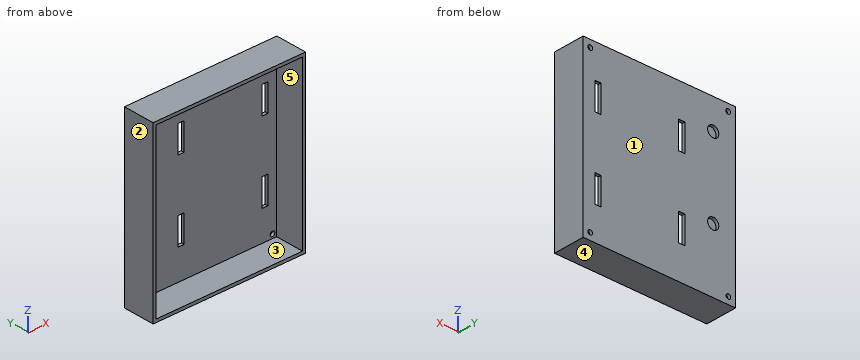
Autodesk Inventor part; units mm, degrees
ref_plane "YZ Plane" through (0, 0, 0) normal (1, 0, 0) x (0, 1, 0)
ref_plane "XZ Plane" through (0, 0, 0) normal (0, 1, 0) x (-1, 0, 0)
ref_plane "XY Plane" through (0, 0, 0) normal (0, 0, 1) x (1, 0, 0)
sketch "Sketch1" plane through (0, 0, 0) normal (0, 1, 0) x (-1, 0, 0)
  line L0 (-58.4836, 42.7915) -> (-27.4836, 42.7915) construction
  line L1 (-27.4836, 42.7915) -> (-27.4836, 11.7915) construction
  line L2 (-27.4836, 11.7915) -> (-58.4836, 11.7915) construction
  line L3 (-58.4836, 11.7915) -> (-58.4836, 20.5915) construction
  line L4 (-58.4836, 42.7915) -> (-27.4836, 11.7915) construction
  line L5 (-27.4836, 42.7915) -> (-58.4836, 11.7915) construction
  line L6 (-58.4836, 3.6103) -> (-27.4836, 3.6103) construction
  line L7 (-27.4836, 3.6103) -> (-27.4836, -27.2085) construction
  line L8 (-27.4836, -27.2085) -> (-58.4836, -27.2085) construction
  line L9 (-58.4836, -27.2085) -> (-58.4836, -18.4991) construction
  line L10 (-58.4836, 3.6103) -> (-27.4836, -27.2085) construction
  line L11 (-20.4336, 38.5415) -> (2.0664, 38.5415) construction
  line L12 (2.0664, 38.5415) -> (2.0664, 16.0415) construction
  line L13 (2.0664, 16.0415) -> (-20.4336, 16.0415) construction
  line L14 (-20.4336, 16.0415) -> (-20.4336, 38.5415) construction
  line L15 (-20.4336, 38.5415) -> (2.0664, 16.0415) construction
  line L16 (2.0664, 38.5415) -> (-20.4336, 16.0415) construction
  line L17 (-20.5481, -0.4585) -> (2.0664, -0.4585) construction
  line L18 (2.0664, -0.4585) -> (2.0664, -22.9585) construction
  line L19 (2.0664, -22.9585) -> (-20.5481, -22.9585) construction
  line L20 (-20.5481, -22.9585) -> (-20.5481, -0.4585) construction
  line L21 (-20.5481, -0.4585) -> (2.0664, -22.9585) construction
  line L22 (2.0664, -0.4585) -> (-20.5481, -22.9585) construction
  line L23 (3.5664, -29.3085) -> (-60.5836, -29.3085) construction
  line L24 (-60.5836, -29.3085) -> (-60.5836, 44.8915) construction
  line L25 (-60.5836, 44.8915) -> (-64.5836, 44.8915) construction
  line L26 (-64.5836, 44.8915) -> (-64.5836, 48.8915)
  line L27 (-64.5836, 48.8915) -> (-60.5836, 48.8915)
  line L28 (-60.5836, 48.8915) -> (-60.5836, 44.8915) construction
  line L29 (-60.5836, -29.3085) -> (-64.5836, -29.3085) construction
  line L30 (-64.5836, -29.3085) -> (-64.5836, -33.3085)
  line L31 (-64.5836, -33.3085) -> (-60.5836, -33.3085)
  line L32 (-60.5836, -33.3085) -> (-60.5836, -29.3085) construction
  line L33 (3.5664, -29.3085) -> (7.5664, -29.3085) construction
  line L34 (7.5664, -29.3085) -> (7.5664, -33.3085)
  line L35 (7.5664, -33.3085) -> (3.5664, -33.3085)
  line L36 (3.5664, -33.3085) -> (3.5664, -29.3085) construction
  line L37 (3.5664, 44.8915) -> (7.5664, 44.8915) construction
  line L38 (7.5664, 44.8915) -> (7.5664, 48.8915)
  line L39 (7.5664, 48.8915) -> (3.5664, 48.8915)
  line L40 (3.5664, 48.8915) -> (3.5664, 44.8915) construction
  circle A0 centre (5.4519, 46.9805) radius 1.15
  circle A1 centre (-62.5836, 46.8915) radius 1.15
  circle A2 centre (-62.5836, -31.3085) radius 1.15
  circle A3 centre (5.5664, -31.3085) radius 1.15
  line L41 (3.5664, 48.8915) -> (-60.5836, 48.8915)
  line L42 (-64.5836, 44.8915) -> (-64.5836, -29.3085)
  line L43 (-60.5836, -33.3085) -> (3.5664, -33.3085)
  line L44 (7.5664, -29.3085) -> (7.5664, 44.8915)
  line L45 (3.5664, 44.8915) -> (-60.5836, 44.8915) construction
  line L46 (3.5664, 44.8915) -> (3.5664, -29.3085) construction
  line L47 (-57.2836, 33.9915) -> (-60.2836, 33.9915)
  line L48 (-60.2836, 33.9915) -> (-60.2836, 20.5915)
  line L49 (-60.2836, 20.5915) -> (-57.2836, 20.5915)
  line L50 (-57.2836, 20.5915) -> (-57.2836, 33.9915)
  line L51 (-57.2836, -5.0991) -> (-60.2836, -5.0991)
  line L52 (-60.2836, -5.0991) -> (-60.2836, -18.4991)
  line L53 (-60.2836, -18.4991) -> (-57.2836, -18.4991)
  line L54 (-57.2836, -18.4991) -> (-57.2836, -5.0991)
  line L55 (-58.4836, 20.5915) -> (-58.4836, 33.9915) construction
  line L56 (-58.4836, 33.9915) -> (-58.4836, 42.7915) construction
  line L57 (-58.4836, -5.0991) -> (-58.4836, 3.6103) construction
  line L58 (-58.4836, -18.4991) -> (-58.4836, -5.0991) construction
  line L59 (-62.5836, 46.8915) -> (-60.5836, 46.8915) construction
  line L60 (-62.5836, 46.8915) -> (-62.5836, 44.8915) construction
  line L61 (-62.5836, 46.8915) -> (-64.5836, 46.8915) construction
  line L62 (-62.5836, 46.8915) -> (-62.5836, 48.8915) construction
  line L63 (-64.5836, -31.3085) -> (-62.5836, -31.3085) construction
  line L64 (-62.5836, -31.3085) -> (-60.5836, -31.3085) construction
  line L65 (-62.5836, -31.3085) -> (-62.5836, -29.3085) construction
  line L66 (-62.5836, -31.3085) -> (-62.5836, -33.3085) construction
  line L67 (5.5664, 46.8915) -> (3.5664, 46.8915) construction
  line L68 (5.5664, 46.8915) -> (7.5664, 46.8915) construction
  line L69 (5.5664, 46.8915) -> (5.5664, 44.8915) construction
  line L70 (5.5664, 44.8915) -> (5.5664, 46.8915) construction
  line L71 (5.5664, 46.8915) -> (5.5664, 48.8915) construction
  line L72 (5.5664, -31.3085) -> (5.5664, -33.3085) construction
  line L73 (5.5664, -31.3085) -> (3.5664, -31.3085) construction
  line L74 (5.5664, -31.3085) -> (5.5664, -29.3085) construction
  line L75 (5.5664, -31.3085) -> (7.5664, -31.3085) construction
  circle A4 centre (-1.9336, 35.5415) radius 2.75
  circle A5 centre (-1.9336, -3.4585) radius 2.75
  line L76 (-1.9336, 35.5415) -> (-1.9336, 38.5415) construction
  line L77 (-1.9336, 35.5415) -> (2.0664, 35.5415) construction
  line L78 (-1.9336, -3.4585) -> (2.0664, -3.4585) construction
  line L79 (-1.9336, -3.4585) -> (-1.9336, -0.4585) construction
  line L80 (-15.9336, 33.9915) -> (-18.9336, 33.9915)
  line L81 (-18.9336, 33.9915) -> (-18.9336, 20.5915)
  line L82 (-18.9336, 20.5915) -> (-15.9336, 20.5915)
  line L83 (-15.9336, 20.5915) -> (-15.9336, 33.9915)
  line L84 (-15.9336, -5.0085) -> (-18.9336, -5.0085)
  line L85 (-18.9336, -5.0085) -> (-18.9336, -18.4085)
  line L86 (-18.9336, -18.4085) -> (-15.9336, -18.4085)
  line L87 (-15.9336, -18.4085) -> (-15.9336, -5.0085)
  line L88 (9.0664, 50.3915) -> (-66.0836, 50.3915)
  line L89 (-66.0836, 50.3915) -> (-66.0836, -34.8085)
  line L90 (-66.0836, -34.8085) -> (9.0664, -34.8085)
  line L91 (9.0664, -34.8085) -> (9.0664, 50.3915)
  point P0 (-89.8981, -75.7195)
  dimension "d0" = 22.5
  dimension "d5" = 31
  dimension "d7" = 22.5
  dimension "d11" = 4
  dimension "d12" = 72.15
  dimension "d13" = 82.2
  dimension "d14" = 2.3
  dimension "d15" = 31
  dimension "d16" = 5.5
  dimension "d17" = 5.5
  dimension "d18" = 10.35
  dimension "d19" = 10.35
  dimension "d20" = 6.1
  dimension "d21" = 6.1
  dimension "d22" = 6.1
  dimension "d23" = 6.1
  dimension "d24" = 3
  dimension "d25" = 13.4
  dimension "d26" = 1.2
  dimension "d27" = 8.1812
  dimension "d28" = 16.5
  dimension "d29" = 5.5
  dimension "d30" = 5.5
  dimension "d31" = 3
  dimension "d32" = 4
  dimension "d33" = 1.5
  dimension "d34" = 4.55
  dimension "d35" = 4.55
  dimension "d36" = 4.55
  dimension "d37" = 1.5
  dimension "d38" = 1.5
  dimension "d39" = 1.5
  dimension "d40" = 1.5
extrude "Edges" add sketch "Sketch1" against normal blind 14 contours L91 L90 L89 L88
extrude "Surface" add sketch "Sketch1" along normal blind 1.5 contours L26 L27 L41 L39 L38 L44 L34 L35 L43 L31 L30 L42 | L91 L90 L89 L88
properties part number "CameraBoardCover" material "NylonD2W"
Design review of the part built by this model. Coordinates are the model's own, in mm. Face numbers are marked on the shaded views. A direction names the side the tool comes from. Coordinates: 2 decimals unless noted, no trailing zeros. Order: outer loops, then holes, each group sorted by start corner. A loop starts at its lowest first (then second) coordinate and runs counter-clockwise, first axis right, second up. Notation, with made-up numbers: (-3.75, 78.25) - (28.25, 78.25) arc R32 cw to (28.25, 106.25) - close; hole circle Ø5 at (-18.5, 74.5). An arc over 180 degrees is marked (long way). Answer in a Markdown table with one row per item.
(1) Clearance check with flat-ended pins moving along their axes: pin 1 (10 mm diameter, centred on x = 19, z = 30, fed in from -Y); pin 2 (3 mm diameter, centred on x = 62.58, z = 46.89, fed in from +Y). State where each tip first meets the part, or that it passes through.
Checked values:
| item | result |
|---|---|
| pin 1 | y = 0 |
| pin 2 | y = 1.5 |
(2) Consider section A-A on z = -2. State the section outline as (x, y) points, plus the area to 3 significant figures.
Checked values:
| item | result |
|---|---|
| outline | (-9.07, -14) - (-7.57, -14) - (-7.57, 0) - (-0.4, 0) - (-0.4, 1.5) - (-9.07, 1.5) - close; (4.26, 0) - (64.58, 0) - (64.58, -14) - (66.08, -14) - (66.08, 1.5) - (4.26, 1.5) - close |
| area | 148 mm^2 |
(3) The part is to be moulded in two halves that separate along X. For the marked faces 1, 2 and 3, say which applies: released by +X, released by -X, zero draft, split by the parting line, or undercut.
Checked values:
| item | result |
|---|---|
| face 1 | zero draft |
| face 2 | released by -X |
| face 3 | undercut |
(4) Wall thickness on line 1 along X through (y, z) = (-10.75, 21.5); line 2 along Z through (x, y) = (-6, -3.5); line 3 along Y through (x, z) = (17, 17.5): over which ranges is each line inside the solid? List them lowest first. Write a range as from..to.
Checked values:
| item | result |
|---|---|
| line 1 | -9.07..-7.57, 64.58..66.08 |
| line 2 | -34.81..-33.31, 48.89..50.39 |
| line 3 | 0..1.5 |
(5) For the marked faces 4 and 5, list the 3-axis set-ups (+Z, -Z, +X, -X, +Y, -Y) from which the entire face can be reached by the end or side of a thin tool; tool diameter is ignored.
Checked values:
| item | result |
|---|---|
| face 4 | -Z, +X, -X, +Y, -Y |
| face 5 | -Y |
(6) Consider section C-C on x = 38. State the section outline as (y, z) points, plus the area to 3 significant figures.
Checked values:
| item | result |
|---|---|
| outline | (-14, -34.81) - (1.5, -34.81) - (1.5, 50.39) - (-14, 50.39) - (-14, 48.89) - (0, 48.89) - (0, -33.31) - (-14, -33.31) - close |
| area | 170 mm^2 |
(7) Consider section B-B on y = -9.25. State the section outline as (x, z) points, plus the area to 3 significant figures.
Checked values:
| item | result |
|---|---|
| outline | (-9.07, -34.81) - (66.08, -34.81) - (66.08, 50.39) - (-9.07, 50.39) - close; hole (-7.57, -33.31) - (64.58, -33.31) - (64.58, 48.89) - (-7.57, 48.89) - close |
| area | 472 mm^2 |
(8) Consider section D-D on z = 12. State the section outline as (x, y) points.
Checked values:
| item | result |
|---|---|
| outline | (-9.07, -14) - (-7.57, -14) - (-7.57, 0) - (64.58, 0) - (64.58, -14) - (66.08, -14) - (66.08, 1.5) - (-9.07, 1.5) - close |
